```python
from build123d import *

# Parameters (mm, degrees)
F1_DEPTH  = 30.734
F3_W      = 32.981223
F3_H      = 10.993741
F4_DEPTH  = 53.848
F5_R      = 9.757889
F6_DEPTH  = 53.086
F8_DEPTH  = 9.906
F9_R      = 1.839631
F11_DEPTH = 10.16
F12_R     = 3.72766
F13_DEPTH = 25.4


with BuildPart() as f1:
    # F0 (on Front) → F1 (new body)
    with BuildSketch(Plane.XZ):
        with BuildLine():
            ThreePointArc((-30.84355, 0.39327), (-19.245074, 5.197517), (-14.440828, 16.795993))
            Line((-14.440828, 16.795993), (-30.84355, 16.795993))
            Line((-30.84355, 16.795993), (-30.84355, 0.39327))
        make_face()
        with BuildLine():
            Line((-30.84355, 16.795993), (-14.440828, 16.795993))
            ThreePointArc((-14.440828, 16.795993), (-42.442027, 28.394469), (-30.84355, 0.39327))
            Line((-30.84355, 0.39327), (-30.84355, 16.795993))
        make_face()
        with BuildLine():
            Line((70.848547, 16.795993), (-14.440828, 16.795993))
            ThreePointArc((-14.440828, 16.795993), (-19.245074, 5.197517), (-30.84355, 0.39327))
            Line((-30.84355, 0.39327), (-30.84355, 0))
            Line((-30.84355, 0), (70.848547, 0))
            Line((70.848547, 0), (70.848547, 16.795993))
        make_face()
    extrude(amount=-F1_DEPTH)

    # F3 (on offset) → F4 (cut)
    with BuildSketch(Plane.XY.offset(34.29)):
        with Locations((-30.843549, 15.269084)):
            Rectangle(F3_W, F3_H)
    extrude(amount=-F4_DEPTH, mode=Mode.SUBTRACT)

    # F5 (on Front) → F6 (cut)
    with BuildSketch(Plane.XZ):
        with Locations((-31.148931, 17.101374)):
            Circle(F5_R)
    extrude(amount=-F6_DEPTH, mode=Mode.SUBTRACT)

    # F7 (on Front) → F8 (join)
    with BuildSketch(Plane.XZ):
        with BuildLine():
            Line((29.622022, 17.101374), (29.622022, 0))
            Line((29.622022, 0), (50.082598, 0))
            Line((50.082598, 0), (50.082598, 34.508131))
            Line((50.082598, 34.508131), (40.921144, 34.508131))
            ThreePointArc((40.921144, 34.508131), (38.063066, 23.992738), (29.622022, 17.101374))
        make_face()
    extrude(amount=-F8_DEPTH)

    # F9
    f9_edges = [f1.edges().sort_by_distance(p)[0] for p in [
        (50.082598, 4.953, 34.508131),
    ]]
    fillet(f9_edges, radius=F9_R)

    # F10 (on Front) → F11 (cut)
    with BuildSketch(Plane.XZ):
        Polygon((29.011261, 0), (29.011261, 17.101374), (7.634541, 16.795993), (16.49061, 0), align=None)
    extrude(amount=-F11_DEPTH, mode=Mode.SUBTRACT)

    # F12 (on face) → F13 (cut)
    with BuildSketch(Plane.XY.offset(16.795993)):
        with Locations((50.387979, 21.987481)):
            Circle(F12_R)
    extrude(amount=-F13_DEPTH, mode=Mode.SUBTRACT)


solid = f1.part
```
Build history of the part. All positions in model axes, mm. A direction names the side the tool comes from. Give positions to 0.01 mm unless a question says otherwise; leave off trailing zeros. Loops run counter-clockwise (first coordinate to the right, second up) from the corner with the lowest first, then second, coordinate; pieces in that order, holes last. Notation, with made-up numbers: (21.5, 8.5) - (29.5, 8.5) arc R28 cw to (29.5, 27.5) - close; hole circle Ø11 at (25, 50.5). An arc over 180 degrees is marked (long way). Use a Markdown table: item, result.
(1) Wall check: line 1 along X through (y, z) = (9, 18); line 2 along X through (y, z) = (3, 21); line 3 along Z through (x, y) = (-9, 28.5). Give the ranges that are in metal, low to high.
Taken from the geometry:
| item | result |
|---|---|
| line 1 | -47.2 to -40.87, -21.43 to -14.49, 31.56 to 50.08 |
| line 2 | -46.7 to -40.09, -22.2 to -14.99, 35.62 to 50.08 |
| line 3 | 0 to 16.8 |
(2) Band-saw the part on C-C (y = 28). Give the cut face in (x, z), and give its area (3 significant figures).
Taken from the geometry:
| item | result |
|---|---|
| outline | (-30.84, 0) - (70.85, 0) - (70.85, 16.8) - (-14.44, 16.8) arc R16.4 ccw (long way) to (-30.84, 0.39) - close; hole circle Ø19.52 at (-31.15, 17.1) |
| area | 2,040 mm2 |
(3) Pull direction X, two halves, no side cores. Call faces 1 (the face through (29.011, 5, 8)), 2 (the face through (50.083, 5, 25)), 3 (the face through (44, 9.906, 24)): +X half, -X half, draft (parallel to the pull), parting line (faces both ways), or undercut.
Taken from the geometry:
| item | result |
|---|---|
| face 1 | undercut |
| face 2 | +X half |
| face 3 | draft |
(4) Which spindle directions (+Z, -Z, +X, -X, +Y, -Y) get a long thin tool onto all of the face, cutting with end or side? Do faces 4 (the face through (-24, 20.766, 9)), 5 (the face through (12, 5.01, 8.52)), 6 (the face through (11, 30.734, 9)). Say none if no direction does.
Taken from the geometry:
| item | result |
|---|---|
| face 4 | +Z, -Z, -X |
| face 5 | +Z, -Y |
| face 6 | +Z, -Z, +X, -X, +Y |
(5) Band-saw the part on A-A (z = 11). Give the cut face in (x, y).
Taken from the geometry:
| item | result |
|---|---|
| outline | (-46.19, 0) - (-38.76, 0) - (-38.76, 9.77) - (-46.19, 9.77) - close; (-46.19, 20.77) - (-38.76, 20.77) - (-38.76, 30.73) - (-46.19, 30.73) - close; (-23.53, 0) - (10.69, 0) - (10.69, 10.16) - (29.01, 10.16) - (29.01, 0) - (70.85, 0) - (70.85, 30.73) - (-23.53, 30.73) - (-23.53, 20.77) - (-14.35, 20.77) - (-14.35, 9.77) - (-23.53, 9.77) - close; hole circle Ø7.46 at (50.39, 21.99) |
(6) Band-saw the part on D-D (z = 19.5). Give the cut face in (x, y), and give its area (3 significant figures).
Taken from the geometry:
| item | result |
|---|---|
| outline | (-47.02, 0) - (-40.61, 0) - (-40.61, 9.77) - (-47.02, 9.77) - close; (-47.02, 20.77) - (-40.61, 20.77) - (-40.61, 30.73) - (-47.02, 30.73) - close; (-21.69, 0) - (-14.67, 0) - (-14.67, 9.77) - (-21.69, 9.77) - close; (-21.69, 20.77) - (-14.67, 20.77) - (-14.67, 30.73) - (-21.69, 30.73) - close; (33.89, 0) - (50.08, 0) - (50.08, 9.91) - (33.89, 9.91) - close |
| area | 426 mm2 |
(7) Band-saw the part on B-B (y = 7). Give the cut face in (x, z).
Taken from the geometry:
| item | result |
|---|---|
| outline | (-30.84, 0) - (16.49, 0) - (7.63, 16.8) - (-14.44, 16.8) arc R16.4 ccw (long way) to (-30.84, 0.39) - close; (29.01, 0) - (70.85, 0) - (70.85, 16.8) - (50.08, 16.8) - (50.08, 32.67) arc R1.84 ccw to (48.24, 34.51) - (40.92, 34.51) arc R17.84 cw to (29.62, 17.1) - (29.62, 16.8) - (29.01, 16.8) - close; hole circle Ø19.52 at (-31.15, 17.1) |
(8) Drop flat-ended pins along their axis: pin 1 Ø9 at (y, z) = (16, 10) entering from -X; pin 2 Ø1.5 at (y, z) = (23.5, 18.5) entering from +X; pin 3 Ø9 at (x, z) = (41.5, 25.5) entering from +Y; pin 4 Ø11.5 at (x, z) = (-31.15, 17.1) entering from +Y. Give the stop position or say it passes through.
Taken from the geometry:
| item | result |
|---|---|
| pin 1 | x = -14.35 |
| pin 2 | x = -14.47 |
| pin 3 | y = 9.91 |
| pin 4 | through |
